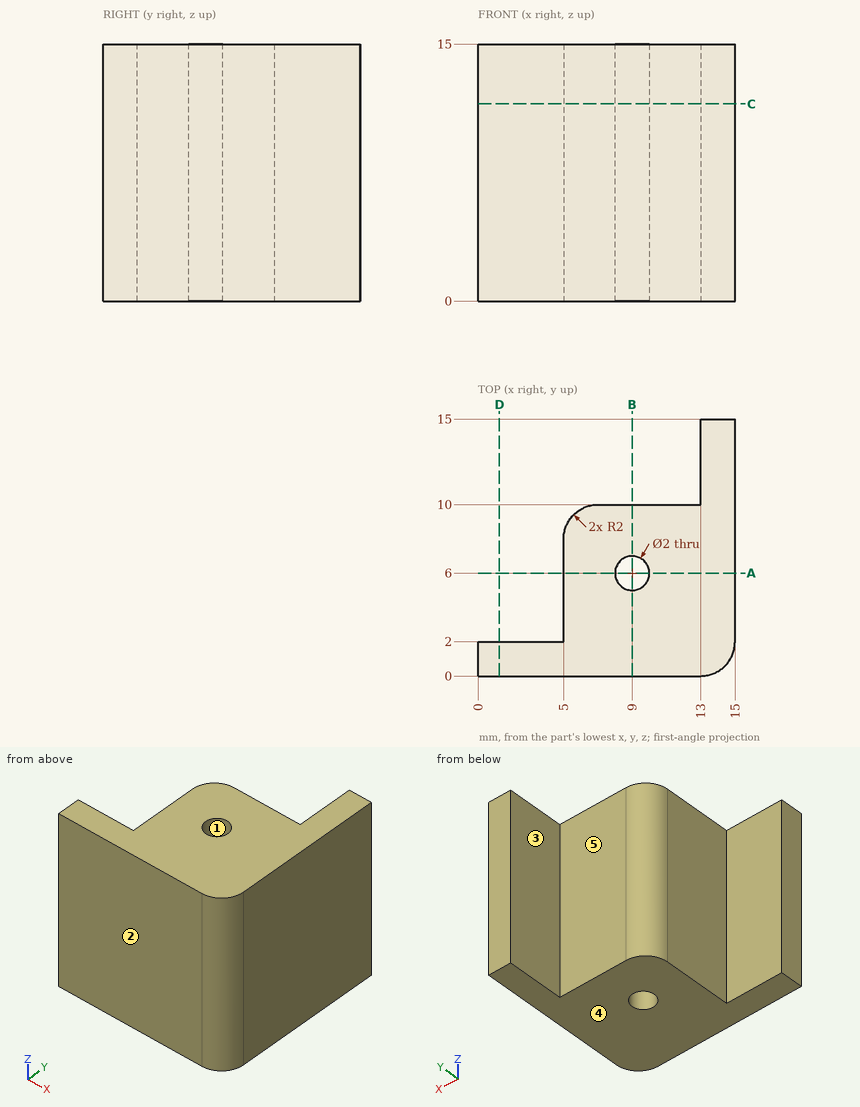
Geometry: see drawing. Coordinates: mm, zero at the bounding-box minimum. A direction names the side the tool comes from. Coordinates: 2 decimals unless noted, no trailing zeros. Order: outer loops, then holes, each group sorted by start corner. A loop starts at its lowest first (then second) coordinate and runs counter-clockwise, first axis right, second up. Notation, with made-up numbers: M 59.5,58.25 L 89.5,58.25 A22 ccw 89.5,94.25 Z; hole C 56.5,-35.5 d3. An arc over 180 degrees is marked long. Answer in a Markdown table with one row per item. Add a question column.
Q1. Section query D-D on x = 1.25. Return the cut outline in (y, z), and give its area (3 significant figures).
Q2. Line query: L1, parallel to Y at x = 9, z = 6; L2, parallel to Y at x = 7.5, z = 0.5; L3, parallel to X at y = 5.5, z = 8.5. Output: solid intervals per line, ascending.
Q3. Section query A-A on y = 6. Return the cut outline in (x, z), and give its area (3 significant figures).
Q4. Contact query for flat-ended pins moving along their axis: P1, Ø3, axis at y = 6.5, z = 7.5, coming from the -X side; P2, Ø4, axis at y = 13.5, z = 6.5, coming from the -X side; P3, Ø6, axis at x = 10.5, z = 10.5, coming from the +Y side; P4, Ø1.6, axis at x = 9, y = 6, coming from the -Z side. Output: stop coordinate, or through.
Q5. Reachability of the marked faces 4 and 5 from +Z, -Z, +X, -X, +Y, -Y: full face, straight path, thin tool, end or side. Return the list, or none.
Q6. Section query B-B on x = 9. Return the cut outline in (y, z), and give its area (3 significant figures).
Q7. Section query C-C on z = 11.5. Return the cut outline in (x, y).
Q8. Mould query, pull axis Y, two halves, no side actions, for the marked faces 1, 2 and 3. Classes: released by +Y, released by -Y, zero draft, split by the parting line, or undercut.
Completed:
| question | item | result |
|---|---|---|
| 1 | outline | M 0,0 L 2,0 L 2,15 L 0,15 Z |
| 1 | area | 30.0 mm2 |
| 2 | L1 | y = 0 to 5, 7 to 10 |
| 2 | L2 | y = 0 to 10 |
| 2 | L3 | x = 5 to 8.13, 9.87 to 15 |
| 3 | outline | M 5,0 L 8,0 L 8,15 L 5,15 Z; M 10,0 L 15,0 L 15,15 L 10,15 Z |
| 3 | area | 120 mm2 |
| 4 | P1 | stops at x = 5 |
| 4 | P2 | stops at x = 13 |
| 4 | P3 | stops at y = 15 |
| 4 | P4 | passes through |
| 5 | face 4 | -Z, +X, -X, +Y, -Y |
| 5 | face 5 | +Z, -Z, -X, +Y |
| 6 | outline | M 0,0 L 5,0 L 5,15 L 0,15 Z; M 7,0 L 10,0 L 10,15 L 7,15 Z |
| 6 | area | 120 mm2 |
| 7 | outline | M 0,0 L 13,0 A2 ccw 15,2 L 15,15 L 13,15 L 13,10 L 7,10 A2 ccw 5,8 L 5,2 L 0,2 Z; hole C 9,6 d2 |
| 8 | face 1 | undercut |
| 8 | face 2 | released by -Y |
| 8 | face 3 | zero draft |
